Can you work these out from the drawing? Everything is in mm from the part's minimum corner. Round coordinates to 2 decimals unless told otherwise and drop trailing zeros. Write each loop counter-clockwise with the first axis right and the second up, starting at its lowest first coordinate (ties: lowest second). Pieces come first, ordered by that corner, then holes.
Q1. I'm going to push flat-ended pins straight in: pin 1 Ø1.2 at (y, z) = (19, 2.5) entering from +X; pin 2 Ø0.8 at (y, z) = (15.5, 2) entering from -X; pin 3 Ø0.5 at (x, y) = (18, 26) entering from +Z. Where does each tip first touch, or does it pass through?
Q2. If we section it at A-A (y = 29): Please give me the cut outline in (x, z), plus the area to 4 significant figures.
Q3. If we section it at B-B (z = 3): Please give me the cut outline in (x, y).
Q4. Please list where these lines run through material, in increasing order: line 1 along X through (y, z) = (7.5, 2.65); line 2 along Z through (x, y) = (1, 7.5).
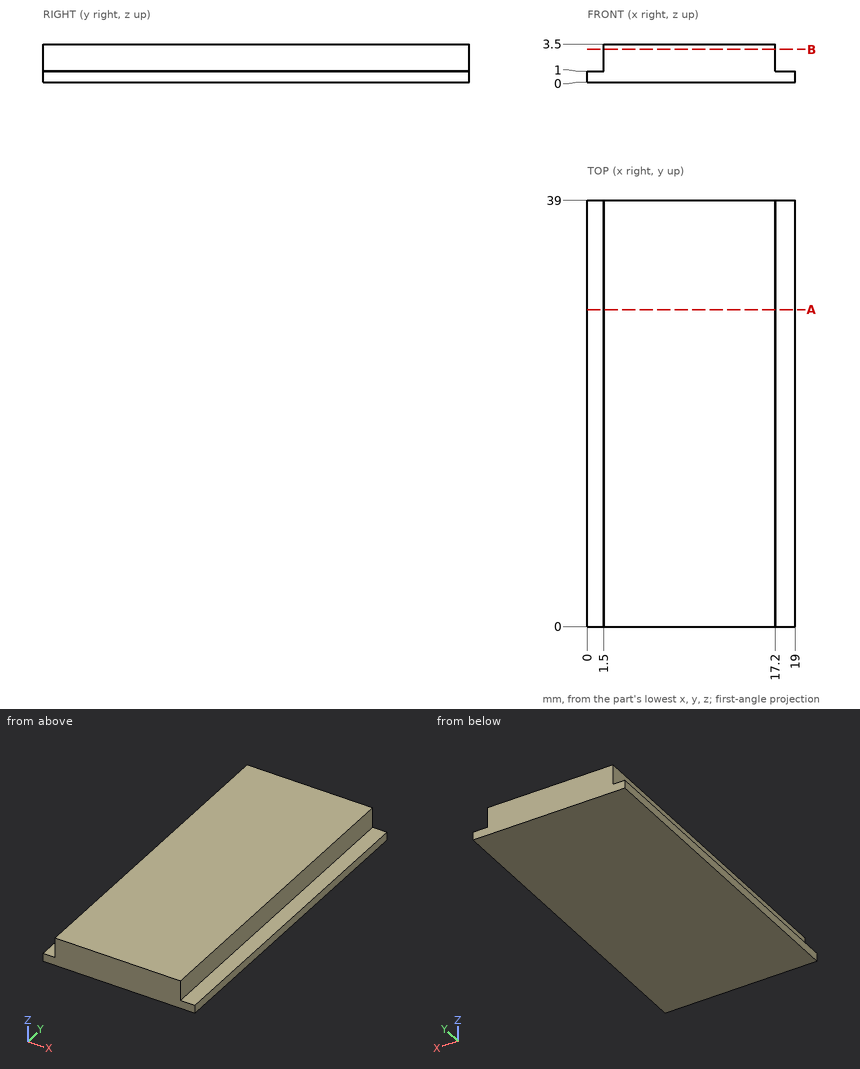
A:
1. pin 1: stops at x = 17.2
1. pin 2: stops at x = 1.5
1. pin 3: stops at z = 1
2. outline: (0, 0) - (19, 0) - (19, 1) - (17.2, 1) - (17.2, 3.5) - (1.5, 3.5) - (1.5, 1) - (0, 1) - close
2. area: 58.25 mm2
3. outline: (1.5, 0) - (17.2, 0) - (17.2, 39) - (1.5, 39) - close
4. line 1: x = 1.5 to 17.2
4. line 2: z = 0 to 1
